Part model, mm, in its own coordinate system. A direction names the side the tool comes from. Give positions to 0.01 mm unless a question says otherwise; leave off trailing zeros. Order: outer loops, then holes, each group sorted by start corner. A loop starts at its lowest first (then second) coordinate and runs counter-clockwise, first axis right, second up. Notation, with made-up numbers: (80, -14.5) - (111, -14.5) arc R15 cw to (111, 4.5) - close; hole circle Ø9 at (-33, -32). An arc over 180 degrees is marked (long way). One line per item, written item: value.
```python
from build123d import *

# Parameters (mm, degrees)
EXTRUDE_1_DEPTH     = 7
SKETCH_2_W          = 7
SKETCH_2_H          = 6
CUT_EXTRUDE_1_DEPTH = 3
SKETCH_3_R          = 1.7
CUT_EXTRUDE_2_DEPTH = 43.178193418
SKETCH_4_W          = 10
SKETCH_4_H          = 5
CUT_EXTRUDE_3_DEPTH = 1


with BuildPart() as part:
    # 草图1 → 凸台-拉伸1 (new body)
    with BuildSketch(Plane.XY):
        Polygon((0, 0), (0, 6), (12, 6), (12, 11), (12, 26), (12, 31), (0, 31), (0, 37), (19, 37), (19, 0), align=None)
    extrude(amount=EXTRUDE_1_DEPTH)

    # 草图2 → 切除-拉伸1 (cut)
    with BuildSketch(Plane(origin=(0, 0, 0), x_dir=(-1, 0, 0), z_dir=(0, 0, -1))):
        with Locations((-15.5, 16.5)):
            Rectangle(SKETCH_2_W, SKETCH_2_H)
    extrude(amount=-CUT_EXTRUDE_1_DEPTH, mode=Mode.SUBTRACT)

    # 草图3 → 切除-拉伸2 (cut, through all)
    with BuildSketch(Plane.ZY):
        with Locations((3, 34)):
            Circle(SKETCH_3_R)
        with Locations((3, 3)):
            Circle(SKETCH_3_R)
    extrude(amount=-CUT_EXTRUDE_2_DEPTH, mode=Mode.SUBTRACT)

    # 草图4 → 切除-拉伸3 (cut)
    with BuildSketch(Plane.XY.offset(7)):
        with Locations((14, 29.5)):
            Rectangle(SKETCH_4_W, SKETCH_4_H)
    extrude(amount=-CUT_EXTRUDE_3_DEPTH, mode=Mode.SUBTRACT)


solid = part.part
```
1) Drill centre lines: line 1 along Y through (x, z) = (5, 3); line 2 along Y through (x, z) = (16.75, 0.5); line 3 along Y through (x, z) = (4, 1.5). Where is each one in solid material? Low to high. Write a range as from..to.
Outcome:
line 1: y = 0..1.3, 4.7..6, 31..32.3, 35.7..37
line 2: y = 0..13.5, 19.5..37
line 3: y = 0..2.2, 3.8..6, 31..33.2, 34.8..37
2) Mould opens along Y. For faces 1 (the flat face through (13.9, 32, 6.5)), 2 (the flat face through (0, 3, 5)), 3 (the flat face through (9, 37, 3)) say: released by +Y, released by -Y, zero draft, split by the parting line, or undercut.
Outcome:
face 1: undercut
face 2: zero draft
face 3: released by +Y
3) Which spindle directions (+Z, -Z, +X, -X, +Y, -Y) get a long thin tool onto all of the face, cutting with end or side? Do faces 4 (the cylindrical face through (9.37, 3.51, 4.62)), 5 (the flat face through (16, 13.5, 1)), 6 (the flat face through (15, 30, 6)), 7 (the flat face through (6, 6, 3)), 8 (the flat face through (15.5, 27, 6.5)). Say none if no direction does.
Outcome:
face 4: +X, -X
face 5: -Z, +X, -X
face 6: +Z, +X
face 7: +Z, -Z, -X
face 8: +Z, +X, -X
4) Cut at C-C, the plane z = 6.5. Give the cut face in (x, y).
Outcome:
outline: (0, 0) - (19, 0) - (19, 27) - (12, 27) - (12, 6) - (0, 6) - close; (0, 31) - (9, 31) - (9, 32) - (19, 32) - (19, 37) - (0, 37) - close
5) Cut at B-B, the plane y = 3. Give the cut face in (x, z), then the cut area to 3 significant figures.
Outcome:
outline: (0, 0) - (19, 0) - (19, 1.3) - (0, 1.3) - close; (0, 4.7) - (19, 4.7) - (19, 7) - (0, 7) - close
area: 68.4 mm^2
6) Cut at D-D, the plane x = 13.5. Give the cut face in (y, z), then the cut area to 3 significant figures.
Outcome:
outline: (0, 0) - (13.5, 0) - (13.5, 3) - (19.5, 3) - (19.5, 0) - (37, 0) - (37, 7) - (32, 7) - (32, 6) - (27, 6) - (27, 7) - (0, 7) - close; hole circle Ø3.4 at (3, 3); hole circle Ø3.4 at (34, 3)
area: 218 mm^2
7) Pin check, flat tips, straight feed: pin 1 (3.5 mm diameter, centred on y = 14.5, z = 4, fed in from -X); pin 2 (3 mm diameter, centred on x = 14.5, y = 16.5, fed in from -Z). Stop position of each tip, or through.
Outcome:
pin 1: stops at x = 12
pin 2: stops at z = 3
8) Cut at A-A, the plane x = 1.75. Give the cut face in (y, z).
Outcome:
outline: (0, 0) - (6, 0) - (6, 7) - (0, 7) - close; (31, 0) - (37, 0) - (37, 7) - (31, 7) - close; hole circle Ø3.4 at (3, 3); hole circle Ø3.4 at (34, 3)
